Geometry: final body of the model. Coordinates: model frame, mm. A direction names the side the tool comes from. Round coordinates to 2 decimals unless told otherwise and drop trailing zeros. Loops run counter-clockwise (first coordinate to the right, second up) from the corner with the lowest first, then second, coordinate; pieces in that order, holes last. Notation, with made-up numbers: M 2.5,-2.75 L 54.5,-2.75 A7 cw 54.5,3.25 Z; hole C -30,42.25 d6. An arc over 180 degrees is marked long. Return JSON: item names as keys, results as strings.
from build123d import *

# Parameters (mm, degrees)
SKETCH1_W           = 400
SKETCH1_H           = 500
BOSS_EXTRUDE1_DEPTH = 20
SKETCH2_W           = 350
SKETCH2_H           = 450
BOSS_EXTRUDE2_DEPTH = 350
CUT_EXTRUDE1_DEPTH  = 320


with BuildPart() as part:
    # Sketch1 → Boss-Extrude1 (new body)
    with BuildSketch(Plane(origin=(0, 0, 0), x_dir=(1, 0, 0), z_dir=(0, 1, 0))):
        Rectangle(SKETCH1_W, SKETCH1_H)
    extrude(amount=-BOSS_EXTRUDE1_DEPTH)

    # Sketch2 → Boss-Extrude2 (add)
    with BuildSketch(Plane.XZ.offset(20)):
        Rectangle(SKETCH2_W, SKETCH2_H)
    extrude(amount=BOSS_EXTRUDE2_DEPTH)

    # Sketch3 → Cut-Extrude1 (cut)
    with BuildSketch(Plane(origin=(175, 0, 0), x_dir=(0, 0, -1), z_dir=(1, 0, 0))):
        Polygon((-185, -50), (185, -50), (185, -100), (165, -100), (165, -120), (185, -120), (185, -170), (-185, -170), (-185, -120), (-165, -120), (-165, -100), (-185, -100), align=None)
        Polygon((-181.478873239, -220), (185, -220), (185, -270), (165, -270), (165, -290), (185, -290), (185, -340), (-181.478873239, -340), (-181.478873239, -290), (-161.478873239, -290), (-161.478873239, -270), (-181.478873239, -270), align=None)
    extrude(amount=-CUT_EXTRUDE1_DEPTH, mode=Mode.SUBTRACT)


solid = part.part
Q1. Section query B-B (z = 172.5). Output: boundary loops of the cut face in (x, y), plus the area to 3 significant figures.
Determined:
{"outline": "M -200,-20 L -175,-20 L -175,-370 L 175,-370 L 175,-340 L -145,-340 L -145,-290 L 175,-290 L 175,-270 L -145,-270 L -145,-220 L 175,-220 L 175,-170 L -145,-170 L -145,-120 L 175,-120 L 175,-100 L -145,-100 L -145,-50 L 175,-50 L 175,-20 L 200,-20 L 200,0 L -200,0 Z", "area": "66,500 mm^2"}
Q2. Pull-direction query (Z, two-part tool) for faces 6 (the flat face through (-3, -10, 250)), 7 (the flat face through (17, -75, -185)), 8 (the flat face through (-200, -10, 3)); classes: pulls with the +Z half, pulls with the -Z half, needs draft (parallel to the pull), parting line crosses it, or undercut.
Determined:
{"face 6": "pulls with the +Z half", "face 7": "undercut", "face 8": "needs draft"}
Q3. Section query C-C (y = -161). Output: boundary loops of the cut face in (x, z), plus the area to 3 significant figures.
Determined:
{"outline": "M -175,-225 L 175,-225 L 175,-185 L -145,-185 L -145,185 L 175,185 L 175,225 L -175,225 Z", "area": "39,100 mm^2"}
Q4. Reachability of faces 1 (the flat face through (-2, -193, -225)), 2 (the flat face through (200, -10, 3)), 3 (the flat face through (-2, -193, 225)), 4 (the flat face through (17, -170, -3)), 5 (the flat face through (-3, 0, -4)) from +Z, -Z, +X, -X, +Y, -Y: full face, straight path, thin tool, end or side. Return the list, or none.
Determined:
{"face 1": "-Z, +X, -X, -Y", "face 2": "+Z, -Z, +X, +Y, -Y", "face 3": "+Z, +X, -X, -Y", "face 4": "+X", "face 5": "+Z, -Z, +X, -X, +Y"}
Q5. Pin query (flat end, axial travel): pin 1 (2 mm diameter, centred on y = -108, z = -111, fed in from +X); pin 2 (5 mm diameter, centred on x = -16.5, y = -140.5, fed in from -Z); pin 3 (25 mm diameter, centred on x = -15.5, y = -64.5, fed in from +Z). Return the tip coordinate at first contact, or that it passes through.
Determined:
{"pin 1": "stops at x = -145", "pin 2": "stops at z = -225", "pin 3": "stops at z = 225"}
Q6. Material intervals for L1, parallel to Y at x = 96.5, z = -6; L2, parallel to Z at x = 30, y = -80.5; L3, parallel to Z at x = 86.5, y = -115, sorted ascending.
Determined:
{"L1": "y = -370 to -340, -220 to -170, -50 to 0", "L2": "z = -225 to -185, 185 to 225", "L3": "z = -225 to -165, 165 to 225"}
Q7. Section query D-D (z = 91.5). Output: boundary loops of the cut face in (x, y).
Determined:
{"outline": "M -200,-20 L -175,-20 L -175,-370 L 175,-370 L 175,-340 L -145,-340 L -145,-220 L 175,-220 L 175,-170 L -145,-170 L -145,-50 L 175,-50 L 175,-20 L 200,-20 L 200,0 L -200,0 Z"}
Q8. Section query A-A (x = 16). State how many separate pieces and enclosed holes the cut face has, plus the area to 3 significant figures.
Determined:
{"separate pieces": "1", "enclosed holes": "2", "area": "80,700 mm^2"}
